Can you work these out from the model? Positions are in its coordinate system, mm. A direction names the side the tool comes from. Round coordinates to 2 decimals unless told otherwise and drop trailing zeros. Loops run counter-clockwise (first coordinate to the right, second up) from the corner with the lowest first, then second, coordinate; pieces in that order, holes last.
(1) I want a section at B-B on y = 1.75. Write out the boundary of the cut face in (x, z), plus the area to 3 significant figures.
(2) If I drill on line 1 along X through (y, z) = (-1.5, 1); line 2 along X through (y, z) = (-1, -23); line 3 along X through (y, z) = (1.5, 3.5), over which ranges is the centre line in solid material (lowest first)?
(3) I want a section at A-A on z = -22.5. Write out the boundary of the cut face in (x, y).
(4) I want a section at C-C on z = 3.5. Write out the boundary of the cut face in (x, y).
(5) Which directions (+Z, -Z, +X, -X, +Y, -Y) give clear straight access to the entire face, cutting with the end or side of a thin tool? Please do faces 1 (the face through (0, 1, -10.25)), 2 (the face through (4.25, 4, 0)), 3 (the face through (24, -1, -9)).
(6) I want a section at D-D on x = -2.5. Write out the boundary of the cut face in (y, z), plus the area to 3 significant figures.
(7) Thinking about a two-plate mould opening in X: for faces 4 (the face through (-4.25, 4, 0)), 5 (the face through (24, -1, -29.75)), 6 (the face through (-24, -1, -9)), which applies, released by +X, released by -X, zero draft, split by the parting line, or undercut?
(8) Will these pins go through, and if not, where does the flat tip stop? pin 1 Ø3 at (y, z) = (2, -17.5) entering from +X; pin 2 Ø5 at (x, z) = (0, -1.5) entering from +Y; pin 3 Ø10 at (x, z) = (12.5, -14.5) entering from -Y; pin 4 Ø5 at (x, y) = (-1, 2.5) entering from -Z.
from build123d import *

# Parameters (mm, degrees)
SKETCH1_W           = 8.5
SKETCH1_H           = 20.5
SKETCH1_W_2         = 6.5
SKETCH1_H_2         = 18.5
EXTRUDE_THIN1_DEPTH = 8
BOSS_EXTRUDE1_DEPTH = 2
CUT_EXTRUDE1_REACH  = 43.729


with BuildPart() as part:
    # Sketch1 → Extrude-Thin1 (new body)
    with BuildSketch(Plane(origin=(0, 0, 0), x_dir=(1, 0, 0), z_dir=(0, 1, 0))):
        Rectangle(SKETCH1_W, SKETCH1_H)
        Rectangle(SKETCH1_W_2, SKETCH1_H_2, mode=Mode.SUBTRACT)
    extrude(amount=EXTRUDE_THIN1_DEPTH)

    # Sketch2 → Boss-Extrude1 (add)
    with BuildSketch(Plane.XZ):
        Polygon((20.5, -29.75), (20.5, -10.25), (-20.5, -10.25), (-20.5, -29.75), (-27.5, -29.75), (-27.5, 10.25), (27.5, 10.25), (27.5, -29.75), align=None)
    extrude(amount=BOSS_EXTRUDE1_DEPTH)

    # Sketch3 → Cut-Extrude1 (cut, up to next)
    with BuildSketch(Plane.XZ.offset(2), mode=Mode.PRIVATE) as cut_extrude1_sk1:
        with BuildLine():
            Line((-24, 8.25), (-24, -27.75))
            ThreePointArc((-24, -27.75), (-24.5, -28.25), (-25, -27.75))
            Line((-25, -27.75), (-25, 8.25))
            ThreePointArc((-25, 8.25), (-24.5, 8.75), (-24, 8.25))
        make_face()
    cut_extrude1_tool1 = extrude(cut_extrude1_sk1.sketch, amount=-CUT_EXTRUDE1_REACH, mode=Mode.PRIVATE) & part.part
    cut_extrude1 = cut_extrude1_tool1.solids().sort_by_distance((-24.5, -2, -9.75))[0]
    add(cut_extrude1, mode=Mode.SUBTRACT)

    # Mirror1: Cut-Extrude1 across plane
    add(cut_extrude1.mirror(Plane(origin=(0, 0, 0), x_dir=(0, 0, 1), z_dir=(1, 0, 0))), mode=Mode.SUBTRACT)


solid = part.part
Filled sheet:
1. outline: (-4.25, -10.25) - (4.25, -10.25) - (4.25, 10.25) - (-4.25, 10.25) - close; hole (-3.25, -9.25) - (3.25, -9.25) - (3.25, 9.25) - (-3.25, 9.25) - close
1. area: 54.0 mm2
2. line 1: x = -27.5 to -25, -24 to 24, 25 to 27.5
2. line 2: x = -27.5 to -25, -24 to -20.5, 20.5 to 24, 25 to 27.5
2. line 3: x = -4.25 to -3.25, 3.25 to 4.25
3. outline: (-27.5, -2) - (-25, -2) - (-25, 0) - (-27.5, 0) - close; (-24, -2) - (-20.5, -2) - (-20.5, 0) - (-24, 0) - close; (20.5, -2) - (24, -2) - (24, 0) - (20.5, 0) - close; (25, -2) - (27.5, -2) - (27.5, 0) - (25, 0) - close
4. outline: (-27.5, -2) - (-25, -2) - (-25, 0) - (-27.5, 0) - close; (-24, -2) - (24, -2) - (24, 0) - (4.25, 0) - (4.25, 8) - (3.25, 8) - (3.25, 0) - (-3.25, 0) - (-3.25, 8) - (-4.25, 8) - (-4.25, 0) - (-24, 0) - close; (25, -2) - (27.5, -2) - (27.5, 0) - (25, 0) - close
5. face 1: -Z, +Y, -Y
5. face 2: +Z, -Z, +X, +Y
5. face 3: +Y, -Y
6. outline: (-2, -10.25) - (8, -10.25) - (8, -9.25) - (0, -9.25) - (0, 9.25) - (8, 9.25) - (8, 10.25) - (-2, 10.25) - close
6. area: 57.0 mm2
7. face 4: released by -X
7. face 5: zero draft
7. face 6: undercut
8. pin 1: passes through
8. pin 2: stops at y = 0
8. pin 3: stops at y = -2
8. pin 4: stops at z = -10.25
